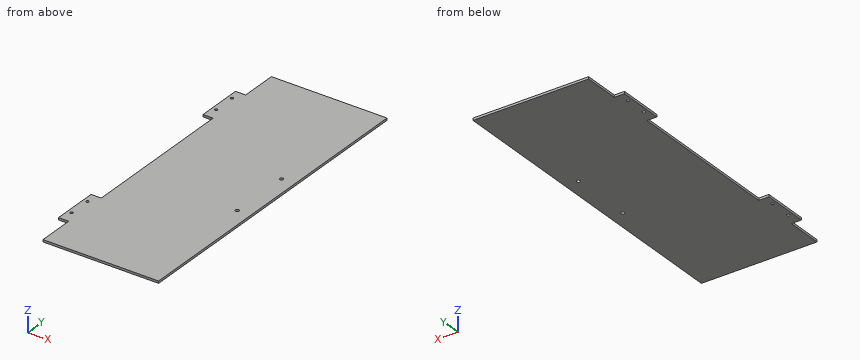
```python
from build123d import *

# Parameters (mm, degrees)
SKETCH1_W           = 164.338
SKETCH1_H           = 458.216
SKETCH1_W_2         = 14.478
SKETCH1_H_2         = 65.278
BOSS_EXTRUDE3_DEPTH = 3.175
SKETCH2_R           = 2.032
CUT_EXTRUDE1_DEPTH  = 4.175
SKETCH4_R           = 2.54
CUT_EXTRUDE3_DEPTH  = 4.175


with BuildPart() as part:
    # Sketch1 → Boss-Extrude3 (new body)
    with BuildSketch(Plane.XY):
        with Locations((-82.169, 229.108)):
            Rectangle(SKETCH1_W, SKETCH1_H)
        with Locations((-171.577, 84.201)):
            Rectangle(SKETCH1_W_2, SKETCH1_H_2)
        with Locations((-171.577, 374.015)):
            Rectangle(SKETCH1_W_2, SKETCH1_H_2)
    extrude(amount=BOSS_EXTRUDE3_DEPTH)

    # Sketch2 → Cut-Extrude1 (cut, through all)
    with BuildSketch(Plane.XY.offset(3.175)):
        with Locations((-172.814936246, 69.493794716)):
            Circle(SKETCH2_R)
        with Locations((-172.814936246, 101.243794716)):
            Circle(SKETCH2_R)
        with Locations((-172.814936246, 391.16)):
            Circle(SKETCH2_R)
        with Locations((-172.814936246, 359.41)):
            Circle(SKETCH2_R)
    extrude(amount=-CUT_EXTRUDE1_DEPTH, mode=Mode.SUBTRACT)

    # Sketch4 → Cut-Extrude3 (cut, through all)
    with BuildSketch(Plane.XY.offset(3.175)):
        with Locations((-19.05, 184.635815808)):
            Circle(SKETCH4_R)
        with Locations((-19.05, 273.535815808)):
            Circle(SKETCH4_R)
    extrude(amount=-CUT_EXTRUDE3_DEPTH, mode=Mode.SUBTRACT)


solid = part.part
```
Check sheet for the modelled part. Datum: model origin and axes. Units: mm. Round coordinates to 2 decimals unless told otherwise and drop trailing zeros. Write each loop counter-clockwise with the first axis right and the second up, starting at its lowest first coordinate (ties: lowest second). Pieces come first, ordered by that corner, then holes. Notation, with made-up numbers: (53.25, 43.5) -> (106.25, 43.5) arc R14 cw to (106.25, 63.5) -> close; hole circle Ø3 at (20.25, -7.75). An arc over 180 degrees is marked (long way). Put each result on its own line as item: value.
(1) Material ranges on line 1 (Y direction, x = -19.05, z = 2.3); line 2 (Y direction, x = -19.5, z = 2.25); line 3 (X direction, y = 359.41, z = 1.9), recorded low to high.
Values found:
line 1: y = 0 to 182.1, 187.18 to 271, 276.08 to 458.22
line 2: y = 0 to 182.14, 187.14 to 271.04, 276.04 to 458.22
line 3: x = -178.82 to -174.85, -170.78 to 0
(2) Go/stop test with flat-tipped pins: pin 1 Ø1 at (y, z) = (435, 1.5) entering from -X; pin 2 Ø1.6 at (x, z) = (-174, 1) entering from +Y; pin 3 Ø2.5 at (x, y) = (-172.81, 101.24) entering from -Z; pin 4 Ø1 at (x, z) = (-174.5, 2) entering from -Y. Record where each tip stops, or that it passes through.
Values found:
pin 1: stops at x = -164.34
pin 2: stops at y = 406.65
pin 3: passes through
pin 4: stops at y = 51.56
(3) Sectioned sample at A-A (z = 1.25). Enter the section's corners in (x, y), plus the area to 3 significant figures.
Values found:
outline: (-178.82, 51.56) -> (-164.34, 51.56) -> (-164.34, 0) -> (0, 0) -> (0, 458.22) -> (-164.34, 458.22) -> (-164.34, 406.65) -> (-178.82, 406.65) -> (-178.82, 341.38) -> (-164.34, 341.38) -> (-164.34, 116.84) -> (-178.82, 116.84) -> close; hole circle Ø4.06 at (-172.81, 69.49); hole circle Ø4.06 at (-172.81, 101.24); hole circle Ø4.06 at (-172.81, 359.41); hole circle Ø4.06 at (-172.81, 391.16); hole circle Ø5.08 at (-19.05, 184.64); hole circle Ø5.08 at (-19.05, 273.54)
area: 77,100 mm^2
(4) Sectioned sample at B-B (y = 257). Enter the section's corners in (x, z) (3 decimals).
Values found:
outline: (-164.338, 0) -> (0, 0) -> (0, 3.175) -> (-164.338, 3.175) -> close
